from build123d import *

# Parameters (mm, degrees)
F0_R      = 25.5
F1_DEPTH  = 2
F0_W      = 200
F0_H      = 170
F0_R_2    = 5
F2_DEPTH  = 5
F0_W_2    = 268
F0_H_2    = 184
F0_W_3    = 208
F0_H_3    = 178
F3_DEPTH  = 160
F4_DEPTH  = 40
F5_R      = 5
F6_DEPTH  = 30.3
F7_DEPTH  = 30
F8_DEPTH  = 10
F9_R      = 10
F10_DEPTH = 30
F11_R     = 20


# Not quite as in the source:
# - a feature names something its author has since deleted; it is built from what else it names


with BuildPart() as f1:
    # F0 (on Top) → F1 (new body)
    with BuildSketch(Plane.XY):
        Circle(F0_R)
    extrude(amount=F1_DEPTH)

    # F0 (on Top) → F2 (join)
    with BuildSketch(Plane.XY):
        with Locations((0, 33)):
            Rectangle(F0_W, F0_H)
        with Locations((-94, 0)):
            Circle(F0_R_2, mode=Mode.SUBTRACT)
        Circle(F0_R, mode=Mode.SUBTRACT)
        with BuildLine():
            Line((94, 10), (94, 0))
            Line((94, 0), (94, -10))
            ThreePointArc((94, -10), (90, -14), (86, -10))
            Line((86, -10), (86, 10))
            ThreePointArc((86, 10), (90, 14), (94, 10))
        make_face(mode=Mode.SUBTRACT)
    extrude(amount=F2_DEPTH)



with BuildPart() as f3:
    # F0 (on Top) → F3 (new body)
    with BuildSketch(Plane.XY):
        with Locations((0, 33)):
            Rectangle(F0_W_2, F0_H_2)
        with Locations((0, 33)):
            Rectangle(F0_W_3, F0_H_3, mode=Mode.SUBTRACT)
    extrude(amount=F3_DEPTH)


with BuildPart() as f1_1:
    add(f1.part)

    add(f3.part)  # F4 merges F3
    # F0 (on Top) → F4 (join)
    with BuildSketch(Plane.XY):
        with Locations((0, 33)):
            Rectangle(F0_W_3, F0_H_3)
        with Locations((0, 33)):
            Rectangle(F0_W, F0_H, mode=Mode.SUBTRACT)
    extrude(amount=F4_DEPTH)

    # F5 (on face) → F6 (cut)
    with BuildSketch(Plane.YZ.offset(134)):
        with Locations((0, 83)):
            Circle(F5_R)
    extrude(amount=-F6_DEPTH, mode=Mode.SUBTRACT)

    # F5 (on face) → F7 (cut)
    with BuildSketch(Plane.YZ.offset(134)):
        with Locations((0, 53)):
            Circle(F5_R)
    extrude(amount=-F7_DEPTH, mode=Mode.SUBTRACT)

    # F0 (on Top) → F8 (cut)
    with BuildSketch(Plane.XY):
        with BuildLine():
            Line((94, -10), (94, 0))
            Line((94, 0), (94, 10))
            ThreePointArc((94, 10), (90, 14), (86, 10))
            Line((86, 10), (86, -10))
            ThreePointArc((86, -10), (90, -14), (94, -10))
        make_face()
    extrude(amount=F8_DEPTH, mode=Mode.SUBTRACT)

    # F9 (on face) → F10 (cut, through all)
    with BuildSketch(Plane(origin=(-134, 0, 0), x_dir=(0, -1, 0), z_dir=(-1, 0, 0))):
        with Locations((-63, 110)):
            Circle(F9_R)
        with Locations((-3, 110)):
            Circle(F9_R)
        with Locations((-63, 50)):
            Circle(F9_R)
        with Locations((-3, 50)):
            Circle(F9_R)
    extrude(amount=-F10_DEPTH, mode=Mode.SUBTRACT)

    # F11
    f11_edges = [f1_1.edges().sort_by_distance(p)[0] for p in [
        (-134, -59, 80),
        (-134, 125, 80),
        (134, 33, 0),
        (134, -59, 80),
        (0, -59, 0),
        (0, 125, 0),
        (-134, 33, 0),
        (134, 125, 80),
    ]]
    fillet(f11_edges, radius=F11_R)


solid = f1_1.part
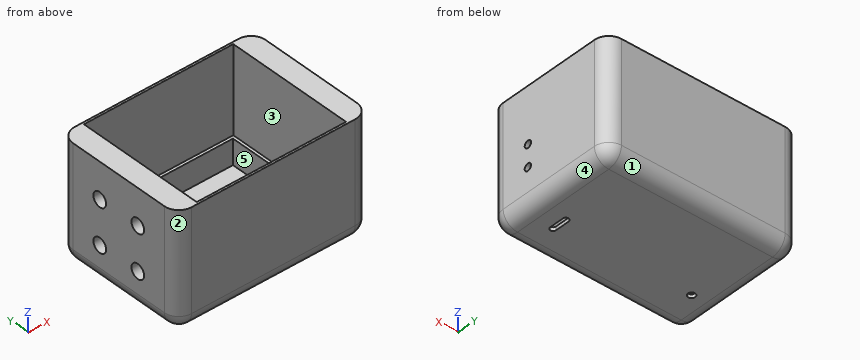
Geometry: final body of the model. Coordinates: model frame, mm. Face numbers are marked on the shaded views. A direction names the side the tool comes from. Coordinates: 2 decimals unless noted, no trailing zeros. Order: outer loops, then holes, each group sorted by start corner. A loop starts at its lowest first (then second) coordinate and runs counter-clockwise, first axis right, second up. Notation, with made-up numbers: (45.5, 19.5) - (62.5, 19.5) arc R13 ccw to (62.5, 41.5) - close; hole circle Ø3 at (-33, 10.5). An arc over 180 degrees is marked (long way). Use one line per item in the form item = value.
1) Section D-D (y = 88). Return loops of the section in (x, z).
Solutions:
outline = (-134, 20) arc R20 ccw to (-114, 0) - (114, 0) arc R20 ccw to (134, 20) - (134, 160) - (104, 160) - (104, 40) - (100, 40) - (100, 5) - (-100, 5) - (-100, 40) - (-104, 40) - (-104, 160) - (-134, 160) - close
2) Set-up query: the marked faces 4 and 5. Return all of +Z, -Z, +X, -X, +Y, -Y with unobstructed straight access to the full face (end or side cutting, diameter ignored); none if empty.
Solutions:
face_4 = -Z, +X, +Y, -Y
face_5 = +Z
3) Section C-C (z = 53). Return loops of the section in (x, y).
Solutions:
outline = (-134, -39) arc R20 ccw to (-114, -59) - (114, -59) arc R20 ccw to (134, -39) - (134, -5) - (104, -5) - (104, -56) - (-104, -56) - (-104, -6.54) - (-134, -6.54) - close; (-134, 12.54) - (-104, 12.54) - (-104, 53.46) - (-134, 53.46) - close; (-134, 72.54) - (-104, 72.54) - (-104, 122) - (104, 122) - (104, 5) - (134, 5) - (134, 105) arc R20 ccw to (114, 125) - (-114, 125) arc R20 ccw to (-134, 105) - close
4) Pin query (flat end, axial travel): pin 1 (1.5 mm diameter, centred on y = 2.5, z = 2.5, fed in from +X); pin 2 (5 mm diameter, centred on x = 4, y = -33, fed in from +Z); pin 3 (2.5 mm diameter, centred on y = -4.5, z = 1.5, fed in from -X). Return the tip coordinate at first contact, or that it passes through.
Solutions:
pin_1 = 124.93
pin_2 = 5
pin_3 = -124.12
5) Mould query, pull axis X, two halves, no side actions, for the marked faces 1, 2 and 3. Classes: +X half, -X half, draft (parallel to the pull), parting line (faces both ways), or undercut.
Solutions:
face_1 = draft
face_2 = -X half
face_3 = undercut
6) Ray query, L1, parallel to X at y = 38.5, z = 108.5; L2, parallel to X at y = 67, z = 31.5; L3, parallel to Y at x = 95, z = 37. Return the intervals inside material, ascending.
Solutions:
L1 = -134 to -104, 104 to 134
L2 = -134 to -100, 100 to 134
L3 = -59 to -52, 118 to 125
7) Section B-B (x = -94). Return loops of the section in (y, z), then the cut area to 3 significant figures.
Solutions:
outline = (-59, 20) arc R20 ccw to (-39, 0) - (-5, 0) - (-5, 5) - (-52, 5) - (-52, 40) - (-56, 40) - (-56, 160) - (-59, 160) - close; (5, 0) - (105, 0) arc R20 ccw to (125, 20) - (125, 160) - (122, 160) - (122, 40) - (118, 40) - (118, 5) - (5, 5) - close
area = 1,910 mm^2
8) Section A-A (z = 104). Return loops of the section in (x, y), then the cut area to 3 significant figures.
Solutions:
outline = (-134, -39) arc R20 ccw to (-114, -59) - (114, -59) arc R20 ccw to (134, -39) - (134, 105) arc R20 ccw to (114, 125) - (-114, 125) arc R20 ccw to (-134, 105) - (-134, 71) - (-104, 71) - (-104, 122) - (104, 122) - (104, -56) - (-104, -56) - (-104, -5) - (-134, -5) - close; (-134, 11) - (-104, 11) - (-104, 55) - (-134, 55) - close
area = 11,000 mm^2
